Geometry: see drawing. Coordinates: mm, zero at the bounding-box minimum. A direction names the side the tool comes from. Give positions to 0.01 mm unless a question says otherwise; leave off trailing zeros. Write each loop counter-clockwise with the first axis right and the second up, starting at its lowest first coordinate (ties: lowest second). Pieces come first, ordered by that corner, then holes. Notation, with made-up numbers: (55, 32.5) - (74, 32.5) arc R12 cw to (74, 38.5) - close; hole circle Ø3 at (73, 89.25). An arc over 180 degrees is marked (long way). Use a Markdown table: item, result. Add a question column.
1. Section query B-B, the plane y = 10. Return loops of the section in (x, z), plus the area to 3 significant figures.
2. Pin query (flat end, axial travel): pin 1 (8 mm diameter, centred on y = 53, z = 58.5, fed in from +X); pin 2 (15 mm diameter, centred on x = 52.5, y = 28.5, fed in from -Z); pin 3 (7.5 mm diameter, centred on y = 44, z = 65.5, fed in from -X). Return the tip coordinate at first contact, or that it passes through.
3. Section query A-A, the plane z = 14. Return loops of the section in (x, y).
4. Section query D-D, the plane x = 39.5. Return loops of the section in (y, z), plus the area to 3 significant figures.
5. Set-up query: the marked faces 4, 5, 6 and 7. Return all of +Z, -Z, +X, -X, +Y, -Y with unobstructed straight access to the full face (end or side cutting, diameter ignored); none if empty.
6. Material intervals for probe 1 along X at (y, z) = (62, 16); probe 2 along Z at (x, y) = (91, 83.5); probe 3 along X at (y, z) = (96.5, 51.5), sorted ascending.
7. Section query C-C, the plane x = 83. Return loops of the section in (y, z).
8. Mould query, pull axis Z, two halves, no side actions, for the marked faces 1, 2 and 3. Classes: released by +Z, released by -Z, zero draft, split by the parting line, or undercut.
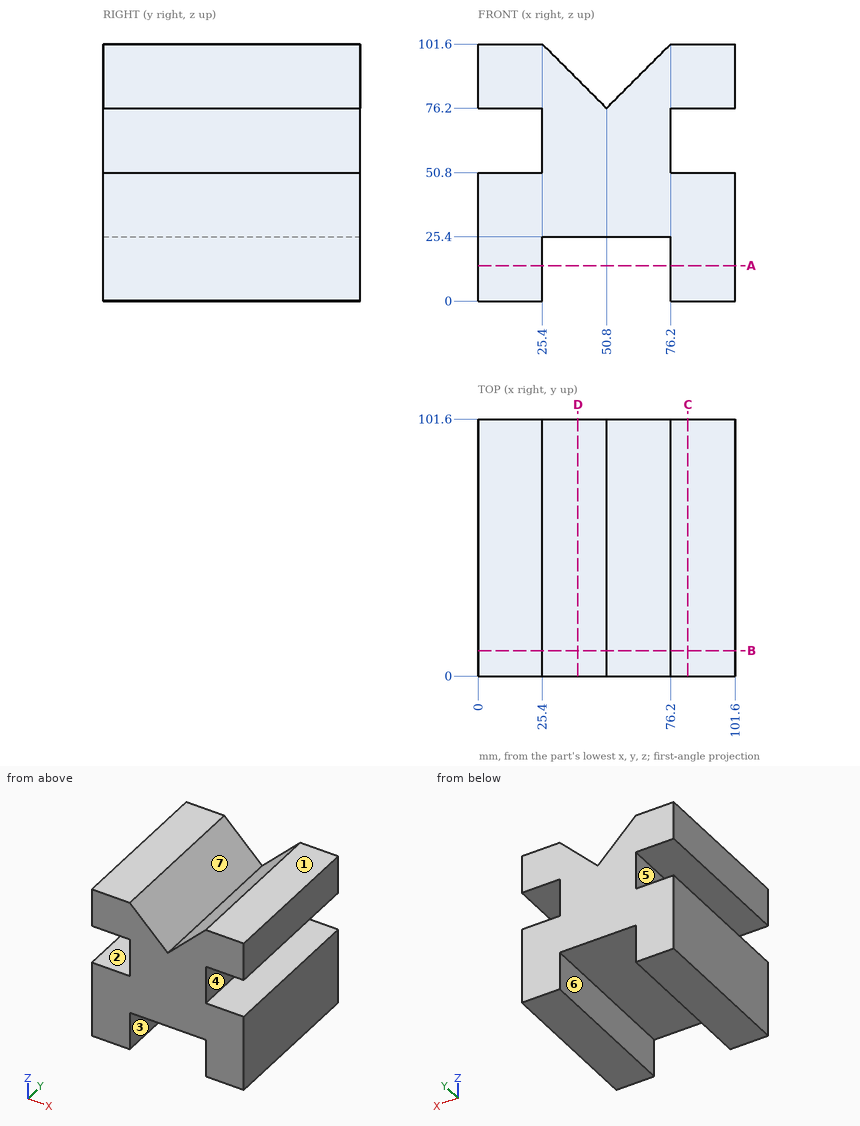
Result sheet:
| question | item | result |
|---|---|---|
| 1 | outline | (0, 0) - (25.4, 0) - (25.4, 25.4) - (76.2, 25.4) - (76.2, 0) - (101.6, 0) - (101.6, 50.8) - (76.2, 50.8) - (76.2, 76.2) - (101.6, 76.2) - (101.6, 101.6) - (76.2, 101.6) - (50.8, 76.2) - (25.4, 101.6) - (0, 101.6) - (0, 76.2) - (25.4, 76.2) - (25.4, 50.8) - (0, 50.8) - close |
| 1 | area | 7,100 mm² |
| 2 | pin 1 | stops at x = 76.2 |
| 2 | pin 2 | stops at z = 25.4 |
| 2 | pin 3 | stops at x = 25.4 |
| 3 | outline | (0, 0) - (25.4, 0) - (25.4, 101.6) - (0, 101.6) - close; (76.2, 0) - (101.6, 0) - (101.6, 101.6) - (76.2, 101.6) - close |
| 4 | outline | (0, 25.4) - (101.6, 25.4) - (101.6, 87.5) - (0, 87.5) - close |
| 4 | area | 6,310 mm² |
| 5 | face 4 | +X, +Y, -Y |
| 5 | face 5 | -X, +Y, -Y |
| 5 | face 6 | -Z, +Y, -Y |
| 5 | face 7 | +Z, +Y, -Y |
| 6 | probe 1 | x = 0 to 25.4, 76.2 to 101.6 |
| 6 | probe 2 | z = 0 to 50.8, 76.2 to 101.6 |
| 6 | probe 3 | x = 25.4 to 76.2 |
| 7 | outline | (0, 0) - (101.6, 0) - (101.6, 50.8) - (0, 50.8) - close; (0, 76.2) - (101.6, 76.2) - (101.6, 101.6) - (0, 101.6) - close |
| 8 | face 1 | released by +Z |
| 8 | face 2 | undercut |
| 8 | face 3 | zero draft |
